Model file for the job. Use its own axes, mm. Face numbers are marked on the shaded views. A direction names the side the tool comes from. Coordinates: 2 decimals unless noted, no trailing zeros. Write each loop counter-clockwise with the first axis right and the second up, starting at its lowest first coordinate (ties: lowest second). Pieces come first, ordered by that corner, then holes. Notation, with made-up numbers: M -14,-4 L 6,-4 A30 cw 6,30 Z; hole C -30,-27.75 d8. An arc over 180 degrees is marked long. Put each result on its own line as item: value. Start each with the question number.
Q1. Cut at C-C (x = 1.2). Write the cut outline in (y, z).
Q2. Cut at B-B (z = 0). Write the cut outline in (x, y), then the cut area to 3 significant figures.
Q3. Cut at D-D (x = -2.2). Write the cut outline in (y, z).
Q4. Drill centre lines: line 1 along X through (y, z) = (6.1, 0); line 2 along Y through (x, z) = (0.9, 2.15); line 3 along Y through (x, z) = (0.15, -0.25). Where is each one in solid material? Low to high.
Q5. Which spindle directions (+Z, -Z, +X, -X, +Y, -Y) get a long thin tool onto all of the face, cutting with end or side? Do the marked faces 4 and 5. Say none if no direction does.
Q6. Cut at A-A (y = 5.5). Write the cut outline in (x, z).
Q7. Pull direction Z, two halves, no side cores. Call the marked faces 1, 2 and 3: pulls with the +Z half, pulls with the -Z half, needs draft (parallel to the pull), parting line crosses it, or undercut.
```python
from build123d import *

# Parameters (mm, degrees)
SALIENTE_EXTRUIR1_DEPTH = 8
CROQUIS2_R              = 1.5
SALIENTE_EXTRUIR2_DEPTH = 6
CROQUIS3_R              = 1.5
CORTAR_EXTRUIR1_DEPTH   = 6


with BuildPart() as part:
    # Croquis1 → Saliente-Extruir1 (new body)
    with BuildSketch(Plane(origin=(0, 0, 0), x_dir=(1, 0, 0), z_dir=(0, 1, 0))):
        Polygon((-2.598076211, 1.5), (-2.598076211, -1.5), (0, -3), (2.598076211, -1.5), (2.598076211, 1.5), (0, 3), align=None)
    extrude(amount=SALIENTE_EXTRUIR1_DEPTH)

    # Croquis2 → Saliente-Extruir2 (add)
    with BuildSketch(Plane.XZ):
        with Locations(Location((0, 0, 0), (0, 0, 270))):
            Circle(CROQUIS2_R)
    extrude(amount=SALIENTE_EXTRUIR2_DEPTH)

    # Croquis3 → Cortar-Extruir1 (cut)
    with BuildSketch(Plane(origin=(0, 8, 0), x_dir=(1, 0, 0), z_dir=(0, 1, 0))):
        with Locations(Location((0, 0, 0), (0, 0, 90))):
            Circle(CROQUIS3_R)
    extrude(amount=-CORTAR_EXTRUIR1_DEPTH, mode=Mode.SUBTRACT)


solid = part.part
```
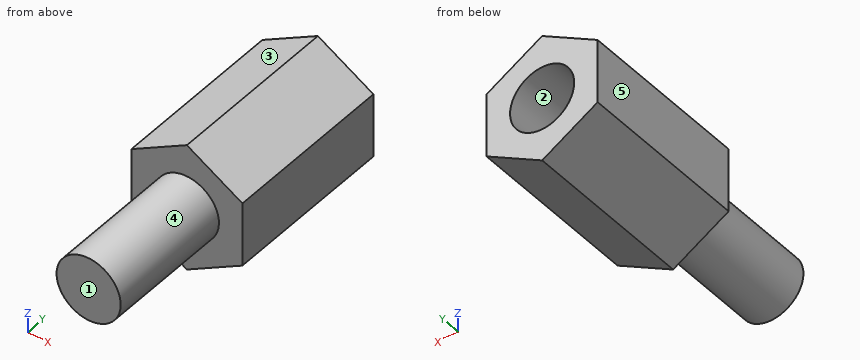
Computed values:
1. outline: M -6,-0.9 L 0,-0.9 L 0,-2.31 L 8,-2.31 L 8,-0.9 L 2,-0.9 L 2,0.9 L 8,0.9 L 8,2.31 L 0,2.31 L 0,0.9 L -6,0.9 Z
2. outline: M -2.6,0 L -1.5,0 L -1.5,-6 L 1.5,-6 L 1.5,0 L 2.6,0 L 2.6,8 L 1.5,8 L 1.5,2 L -1.5,2 L -1.5,8 L -2.6,8 Z
2. area: 41.6 mm2
3. outline: M 0,-1.73 L 8,-1.73 L 8,1.73 L 0,1.73 Z
4. line 1: -2.6 to -1.5, 1.5 to 2.6
4. line 2: 0 to 8
4. line 3: -6 to 2
5. face 4: -Y
5. face 5: +Z, -Z, -X, +Y, -Y
6. outline: M -2.6,-1.5 L 0,-3 L 2.6,-1.5 L 2.6,1.5 L 0,3 L -2.6,1.5 Z; hole C 0,0 d3
7. face 1: needs draft
7. face 2: undercut
7. face 3: pulls with the +Z half
